Print and shaded views of the part. All mm, measured from the part's lowest x, y and z. Coordinates: 2 decimals unless noted, no trailing zeros. Loops run counter-clockwise (first coordinate to the right, second up) from the corner with the lowest first, then second, coordinate; pieces in that order, holes last.
1) Saw through at D-D, the plane z = 2.15. Write the cut outline in (x, y).
2) Two-plate mould, pull along Y, no slides. Class the marked faces 1, 2, 3 and 4: +Y half, -Y half, draft (parallel to the pull), parting line (faces both ways), or undercut.
3) Pin check, flat tips, straight feed: pin 1 Ø4 at (x, y) = (9.5, 8) entering from +Z; pin 2 Ø3.5 at (x, y) = (4, 18.5) entering from +Z. Stop position of each tip, or through.
4) Wall check: line 1 along X through (y, z) = (14.35, 2); line 2 along Y through (x, z) = (5.6, 1.75); line 3 along Z through (x, y) = (8.5, 14.5). Give the ranges that are in metal, low to high.
5) Saw through at C-C, the plane y = 14.35. Write the cut outline in (x, z).
6) Saw through at B-B, the plane z = 4.25. Write the cut outline in (x, y).
7) Saw through at A-A, the plane x = 5.6. Write the cut outline in (y, z), and give its area (3 significant figures).
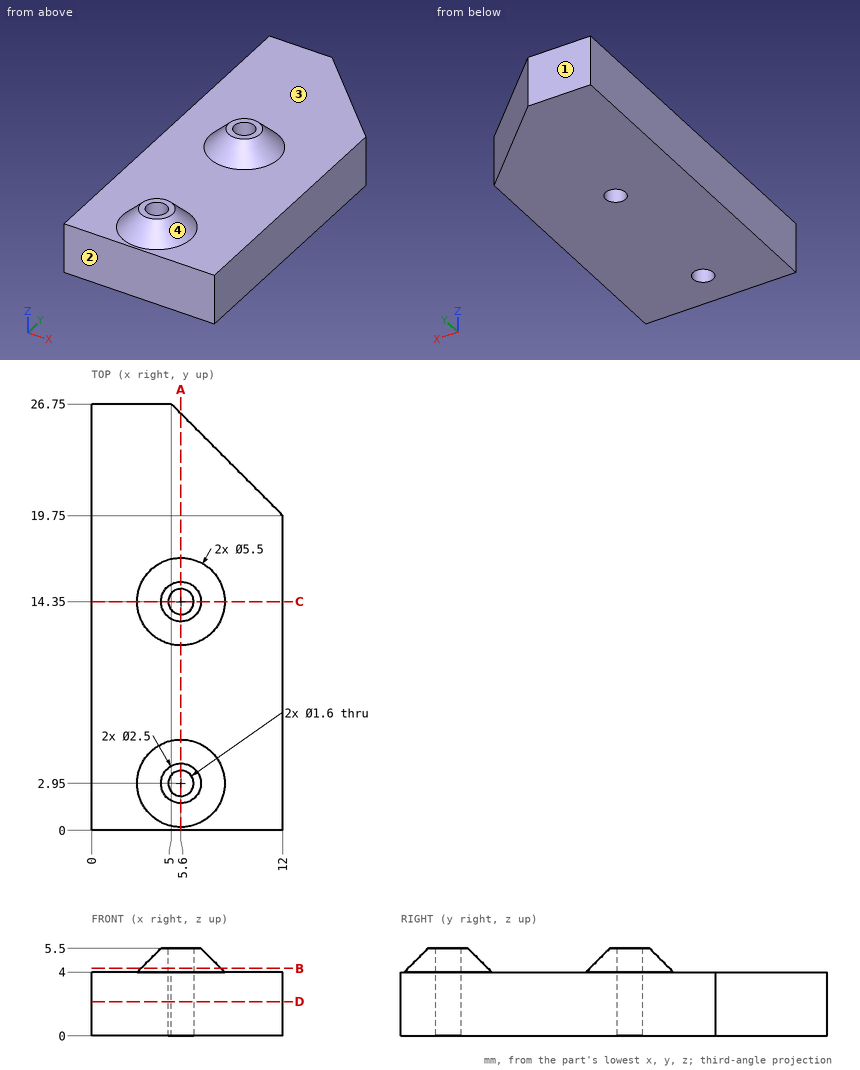
Data:
1. outline: (0, 0) - (12, 0) - (12, 19.75) - (5, 26.75) - (0, 26.75) - close; hole circle Ø1.6 at (5.6, 2.95); hole circle Ø1.6 at (5.6, 14.35)
2. face 1: +Y half
2. face 2: -Y half
2. face 3: undercut
2. face 4: undercut
3. pin 1: stops at z = 4
3. pin 2: stops at z = 4.05
4. line 1: x = 0 to 4.8, 6.4 to 12
4. line 2: y = 0 to 2.15, 3.75 to 13.55, 15.15 to 26.15
4. line 3: z = 0 to 4
5. outline: (0, 0) - (4.8, 0) - (4.8, 5.5) - (4.35, 5.5) - (2.85, 4) - (0, 4) - close; (6.4, 0) - (12, 0) - (12, 4) - (8.35, 4) - (6.85, 5.5) - (6.4, 5.5) - close
6. outline: circle Ø5 at (5.6, 2.95); circle Ø5 at (5.6, 14.35); hole circle Ø1.6 at (5.6, 2.95); hole circle Ø1.6 at (5.6, 14.35)
7. outline: (0, 0) - (2.15, 0) - (2.15, 5.5) - (1.7, 5.5) - (0.2, 4) - (0, 4) - close; (3.75, 0) - (13.55, 0) - (13.55, 5.5) - (13.1, 5.5) - (11.6, 4) - (5.7, 4) - (4.2, 5.5) - (3.75, 5.5) - close; (15.15, 0) - (26.15, 0) - (26.15, 4) - (17.1, 4) - (15.6, 5.5) - (15.15, 5.5) - close
7. area: 99.0 mm2
